Here's how the part is built. I have some questions about the finished solid (model axes, mm). A direction names the side the tool comes from. Round coordinates to 2 decimals unless told otherwise and drop trailing zeros. Loops run counter-clockwise (first coordinate to the right, second up) from the corner with the lowest first, then second, coordinate; pieces in that order, holes last. Notation, with made-up numbers: (7.5, 14) - (41.5, 14) arc R4 ccw to (41.5, 19) - close; hole circle Ø3 at (42.25, 5). An arc over 180 degrees is marked (long way). Answer as a JSON object with one key per item and string values. Group by question number.
1) If we mould it in two halves opening along Z, with no side actions, what happens to faces 4 (the face through (20, 0, 0)), 5 (the face through (4, 0, 12.5)), 6 (the face through (4.96, -7.88, 2.34)), 7 (the face through (0, 4, -3))? For each: pulls with the +Z half, pulls with the -Z half, needs draft (parallel to the pull), parting line crosses it, or undercut.
2) If I drill on line 1 along Z through (x, y) = (-1, -7.75); line 2 along Y through (x, z) = (7, -3); line 3 along Y through (x, z) = (14, 3), over which ranges is the centre line in solid material (lowest first)? Write a range as [from, to].
3) I want a section at B-B, the plane x = 17.5. Please give me the cut outline in (y, z).
4) I want a section at C-C, the plane x = -1. Please give me the cut outline in (y, z), then the cut area to 3 significant figures.
5) Which directions (+Z, -Z, +X, -X, +Y, -Y) give clear straight access to the entire face, cutting with the end or side of a thin tool? Please do faces 1 (the face through (4, 0, -12.5)), 2 (the face through (-2.204, -20.825, -4.962)), 3 (the face through (9.86, 2.131, -1.214)).
6) I want a section at A-A, the plane y = 3.5. Please give me the cut outline in (x, z), then the cut area to 3 significant figures.
7) I want a section at D-D, the plane z = -9. Please give me the cut outline in (x, y).
8) Will these pins go through, and if not, where does the flat tip stop? P1, Ø1.3, axis at y = 4, z = -2, coming from the +X side; P2, Ø8, axis at y = -25.5, z = -0.5, coming from the +X side; P3, Ø4, axis at x = 17, z = -6.5, coming from the -Y side.
from build123d import *

# Parameters (mm, degrees)
SKETCH1_W           = 25
SKETCH1_H           = 14
SKETCH1_R           = 2.25
BOSS_EXTRUDE1_DEPTH = 20
SKETCH2_W           = 25
SKETCH2_H           = 14
BOSS_EXTRUDE2_DEPTH = 12
SKETCH3_R           = 11
BOSS_EXTRUDE3_DEPTH = 1.5
SKETCH4_R           = 10
SKETCH4_R_2         = 6.25
CUT_EXTRUDE1_DEPTH  = 1.25
SKETCH5_R           = 5.55625
BOSS_EXTRUDE4_DEPTH = 26
CHAMFER1_SIZE       = 1
CHAMFER1_SIZE2      = 0.577350269


with BuildPart() as part:
    # Sketch1 → Boss-Extrude1 (new body)
    with BuildSketch(Plane(origin=(0, 0, 0), x_dir=(0, 0, -1), z_dir=(1, 0, 0))):
        Rectangle(SKETCH1_W, SKETCH1_H)
        with Locations((8.5, -1)):
            Circle(SKETCH1_R, mode=Mode.SUBTRACT)
        with Locations((3, 3.5)):
            Circle(SKETCH1_R, mode=Mode.SUBTRACT)
        with Locations((-3, 3.5)):
            Circle(SKETCH1_R, mode=Mode.SUBTRACT)
        with Locations((-9, 3.5)):
            Circle(SKETCH1_R, mode=Mode.SUBTRACT)
    extrude(amount=BOSS_EXTRUDE1_DEPTH)

    # Sketch2 → Boss-Extrude2 (add)
    with BuildSketch(Plane.ZY):
        Rectangle(SKETCH2_W, SKETCH2_H)
    extrude(amount=BOSS_EXTRUDE2_DEPTH)

    # Sketch3 → Boss-Extrude3 (add)
    with BuildSketch(Plane.XZ.offset(7)):
        with Locations((-1, 0)):
            Circle(SKETCH3_R)
    extrude(amount=BOSS_EXTRUDE3_DEPTH)

    # Sketch4 → Cut-Extrude1 (cut)
    with BuildSketch(Plane.XZ.offset(8.5)):
        with Locations((-1, 0)):
            Circle(SKETCH4_R)
        with Locations((-1, 0.461771611)):
            Circle(SKETCH4_R_2, mode=Mode.SUBTRACT)
    extrude(amount=-CUT_EXTRUDE1_DEPTH, mode=Mode.SUBTRACT)

    # Sketch5 → Boss-Extrude4 (add)
    with BuildSketch(Plane.XZ.offset(8.5)):
        with Locations((-1, 0.461771611)):
            Circle(SKETCH5_R)
    extrude(amount=BOSS_EXTRUDE4_DEPTH)

    # Chamfer1
    chamfer1_edges = [part.edges().sort_by_distance(p)[0] for p in [
        (-6.55625, -34.5, 0.461771611),
    ]]
    chamfer1_side = [part.faces().sort_by_distance(p)[0] for p in [
        (-6.55625, -21.5, 0.461771611),
    ]]
    chamfer(chamfer1_edges, length=CHAMFER1_SIZE, length2=CHAMFER1_SIZE2, reference=chamfer1_side[0])


solid = part.part
Outcome:
{
 "1": {"face 4": "needs draft", "face 5": "pulls with the +Z half", "face 6": "undercut", "face 7": "undercut"},
 "2": {"line 1": "[-11, -10], [-5.79, 6.71], [10, 11]", "line 2": "[-7.25, 1.25], [5.75, 7]", "line 3": "[-7, 1.25], [5.75, 7]"},
 "3": {"outline": "(-7, -12.5) - (7, -12.5) - (7, 12.5) - (-7, 12.5) - close; hole circle Ø4.5 at (-1, -8.5); hole circle Ø4.5 at (3.5, -3); hole circle Ø4.5 at (3.5, 3); hole circle Ø4.5 at (3.5, 9)"},
 "4": {"outline": "(-34.5, -4.52) - (-33.5, -5.09) - (-8.5, -5.09) - (-8.5, -5.79) - (-7.25, -5.79) - (-7.25, -10) - (-8.5, -10) - (-8.5, -11) - (-7, -11) - (-7, -12.5) - (7, -12.5) - (7, 12.5) - (-7, 12.5) - (-7, 11) - (-8.5, 11) - (-8.5, 10) - (-7.25, 10) - (-7.25, 6.71) - (-8.5, 6.71) - (-8.5, 6.02) - (-33.5, 6.02) - (-34.5, 5.44) - close", "area": "662 mm^2"},
 "5": {"face 1": "-Z, +X, -X, +Y, -Y", "face 2": "-Y", "face 3": "+X"},
 "6": {"outline": "(-12, -12.5) - (20, -12.5) - (20, -5.25) - (0, -5.25) - (0, -0.75) - (20, -0.75) - (20, 0.75) - (0, 0.75) - (0, 5.25) - (20, 5.25) - (20, 6.75) - (0, 6.75) - (0, 11.25) - (20, 11.25) - (20, 12.5) - (-12, 12.5) - close", "area": "530 mm^2"},
 "7": {"outline": "(-12, -7) - (-7.32, -7) - (-7.32, -8.5) - (-5.36, -8.5) - (-5.36, -7.25) - (3.36, -7.25) - (3.36, -8.5) - (5.32, -8.5) - (5.32, -7) - (20, -7) - (20, -3.19) - (0, -3.19) - (0, 1.19) - (20, 1.19) - (20, 7) - (-12, 7) - close"},
 "8": {"P1": "x = 0", "P2": "x = 4.56", "P3": "y = -7"}
}
